from build123d import *

# Parameters (mm, degrees)
SKETCH2_R           = 45.212
SKETCH2_R_2         = 32.258
BOSS_EXTRUDE3_DEPTH = 40.64
SKETCH4_R           = 32.258
BOSS_EXTRUDE4_DEPTH = 7.62
BOSS_EXTRUDE4_TAPER = 25
CUT_EXTRUDE1_DEPTH  = 81.10791158
SKETCH7_R           = 2.286
CUT_EXTRUDE2_DEPTH  = 81.107911519
BOSS_EXTRUDE8_START = -7.62
BOSS_EXTRUDE8_DEPTH = 11.684
SKETCH18_R          = 8.567257543
CUT_EXTRUDE3_DEPTH  = 5.08
SKETCH19_R          = 2.286
CUT_EXTRUDE4_DEPTH  = 85.454467418
BOSS_EXTRUDE9_START = -15.24
BOSS_EXTRUDE9_DEPTH = 15.24
CUT_EXTRUDE5_START  = -28.956
SKETCH21_R          = 2.286
CUT_EXTRUDE5_DEPTH  = 28.956
CIRPATTERN1_COUNT   = 2


with BuildPart() as part:
    # Sketch2 → Boss-Extrude3 (new body)
    # profile 1 of 2: a face of its own
    with BuildSketch(Plane(origin=(0, 0, 0), x_dir=(1, 0, 0), z_dir=(0, 1, 0))):
        with Locations(Location((0, 0, 0), (0, 0, 270))):
            Circle(SKETCH2_R)
        Circle(SKETCH2_R_2, mode=Mode.SUBTRACT)
    # profile 2 of 2: a face of its own
    with BuildSketch(Plane(origin=(0, 0, 0), x_dir=(1, 0, 0), z_dir=(0, 1, 0))):
        Circle(SKETCH2_R_2)
        Polygon((0, 6.35), (-6.35, 3.483506942), (-6.35, -3.483506942), (0, -6.35), (6.35, -3.483506942), (6.35, 3.483506942), align=None, mode=Mode.SUBTRACT)
    extrude(amount=-BOSS_EXTRUDE3_DEPTH)

    # Sketch4 → Boss-Extrude4 (add)
    with BuildSketch(Plane(origin=(0, 0, 0), x_dir=(1, 0, 0), z_dir=(0, 1, 0))):
        Circle(SKETCH4_R)
    extrude(amount=BOSS_EXTRUDE4_DEPTH, taper=BOSS_EXTRUDE4_TAPER)

    # Sketch6 → Cut-Extrude1 (cut, through all)
    with BuildSketch(Plane(origin=(0, -40.64, 0), x_dir=(-1, 0, 0), z_dir=(0, -1, 0))):
        Polygon((6.35, -3.483506942), (0, -6.35), (-6.35, -3.483506942), (-6.35, 3.483506942), (0, 6.35), (6.35, 3.483506942), align=None)
    extrude(amount=-CUT_EXTRUDE1_DEPTH, mode=Mode.SUBTRACT)

    # Sketch7 → Cut-Extrude2 (cut, through all)
    with BuildSketch(Plane(origin=(0, 7.62, 0), x_dir=(1, 0, 0), z_dir=(0, 1, 0))):
        with Locations(Location((-16.495222192, 16.6624, 0), (0, 0, 270))):
            Circle(SKETCH7_R)
        with Locations(Location((16.6624, 16.6624, 0), (0, 0, 270))):
            Circle(SKETCH7_R)
        with Locations(Location((16.6624, -16.6624, 0), (0, 0, 270))):
            Circle(SKETCH7_R)
        with Locations(Location((-16.495222192, -16.6624, 0), (0, 0, 270))):
            Circle(SKETCH7_R)
    extrude(amount=-CUT_EXTRUDE2_DEPTH, mode=Mode.SUBTRACT)

    # Sketch12 → Boss-Extrude8 (add)
    with BuildSketch(Plane(origin=(0, 7.62, 0), x_dir=(1, 0, 0), z_dir=(0, 1, 0)).offset(BOSS_EXTRUDE8_START)):
        with BuildLine():
            ThreePointArc((-45.091998917, -3.291895759), (-45.888251869, -5.330050438), (-47.973633707, -5.992829324))
            ThreePointArc((-47.973633707, -5.992829324), (-61.102572974, -22.2395178), (-40.602051954, -26.246083736))
            ThreePointArc((-40.602051954, -26.246083736), (-38.578530729, -25.413344212), (-36.658465006, -26.462839746))
            ThreePointArc((-36.658465006, -26.462839746), (-42.485382771, -15.46341472), (-45.091998917, -3.291895759))
        make_face()
    extrude(amount=-BOSS_EXTRUDE8_DEPTH)

    # Sketch18 → Cut-Extrude3 (cut)
    with BuildSketch(Plane(origin=(0, 0, 0), x_dir=(1, 0, 0), z_dir=(0, 1, 0))):
        with Locations(Location((-49.645840541, -18.069608212, 0), (0, 0, 270))):
            Circle(SKETCH18_R)
    extrude(amount=-CUT_EXTRUDE3_DEPTH, mode=Mode.SUBTRACT)

    # Sketch19 → Cut-Extrude4 (cut, through all)
    with BuildSketch(Plane(origin=(0, -5.08, 0), x_dir=(1, 0, 0), z_dir=(0, 1, 0))):
        with Locations(Location((-49.645840541, -18.069608212, 0), (0, 0, 270))):
            Circle(SKETCH19_R)
    extrude(amount=-CUT_EXTRUDE4_DEPTH, mode=Mode.SUBTRACT)

    # Sketch20 → Boss-Extrude9 (add)
    with BuildSketch(Plane.XZ.offset(40.64).offset(BOSS_EXTRUDE9_START)):
        with BuildLine():
            ThreePointArc((42.485382852, -15.463414497), (44.831385262, -12.89196184), (48.307822394, -12.717373918))
            Line((48.307822394, -12.717373918), (61.237093085, -17.295868799))
            Line((61.237093085, -17.295868799), (62.000175566, -15.140990351))
            Line((62.000175566, -15.140990351), (60.601893265, -12.209430544))
            Line((60.601893265, -12.209430544), (44.72934622, -6.588666841))
            ThreePointArc((44.72934622, -6.588666841), (43.832551012, -11.082978649), (42.485382852, -15.463414497))
        make_face()
        with BuildLine():
            ThreePointArc((45.180509286, -21.309596065), (42.629626793, -18.941243028), (42.485382852, -15.463414497))
            ThreePointArc((42.485382852, -15.463414497), (40.701683588, -19.684966271), (38.499780526, -23.704257918))
            Line((38.499780526, -23.704257918), (54.271814253, -29.601179693))
            Line((54.271814253, -29.601179693), (57.22733096, -28.254273131))
            Line((57.22733096, -28.254273131), (58.027905034, -26.113040506))
            Line((58.027905034, -26.113040506), (45.180509286, -21.309596065))
        make_face()
    extrude(amount=BOSS_EXTRUDE9_DEPTH)

    # Sketch21 → Cut-Extrude5 (cut)
    # profile 1 of 2: a face of its own
    with BuildSketch(Plane.XZ.offset(40.64).offset(CUT_EXTRUDE5_START)):
        with BuildLine():
            Line((-20.08732464, 27.438707345), (-28.082012675, 35.43339538))
            ThreePointArc((-28.082012675, 35.43339538), (-31.885487137, 32.053715136), (-35.285134805, 28.268077504))
            Line((-35.285134805, 28.268077504), (-27.271504992, 20.254502449))
            Line((-27.271504992, 20.254502449), (-30.86360744, 16.662375455))
            Line((-30.86360744, 16.662375455), (-23.679427089, 9.478195103))
            ThreePointArc((-23.679427089, 9.478195103), (-9.311017295, 9.478195103), (-9.311017295, 23.846604897))
            Line((-9.311017295, 23.846604897), (-16.495222192, 31.030809794))
            Line((-16.495222192, 31.030809794), (-20.08732464, 27.438707345))
        make_face()
        with Locations(Location((-16.495222192, 16.6624, 0), (0, 0, 90))):
            Circle(SKETCH21_R, mode=Mode.SUBTRACT)
    # profile 2 of 2: a face of its own
    with BuildSketch(Plane.XZ.offset(40.64).offset(CUT_EXTRUDE5_START)):
        with BuildLine():
            ThreePointArc((16.6624, 26.8224), (6.5024, 16.6624), (16.6624, 6.5024))
            Line((16.6624, 6.5024), (26.8224, 6.5024))
            Line((26.8224, 6.5024), (26.8224, 11.844066963))
            Line((26.8224, 11.844066963), (43.63304965, 11.844066963))
            ThreePointArc((43.63304965, 11.844066963), (41.873887087, 17.050000709), (39.496151472, 22.004066963))
            Line((39.496151472, 22.004066963), (25.304864582, 22.004066963))
            Line((25.304864582, 22.004066963), (25.304864582, 26.8224))
            Line((25.304864582, 26.8224), (16.6624, 26.8224))
        make_face()
        with Locations(Location((16.6624, 16.6624, 0), (0, 0, 90))):
            Circle(SKETCH21_R, mode=Mode.SUBTRACT)
    cut_extrude5 = extrude(amount=CUT_EXTRUDE5_DEPTH, mode=Mode.SUBTRACT)

    # CirPattern1: Cut-Extrude5 ×2 about axis
    cirpattern1_axis = Axis((0, 0, 0), (0, 1, 0))
    for i in range(1, CIRPATTERN1_COUNT):
        add(cut_extrude5.rotate(cirpattern1_axis, i * 360 / CIRPATTERN1_COUNT), mode=Mode.SUBTRACT)


solid = part.part
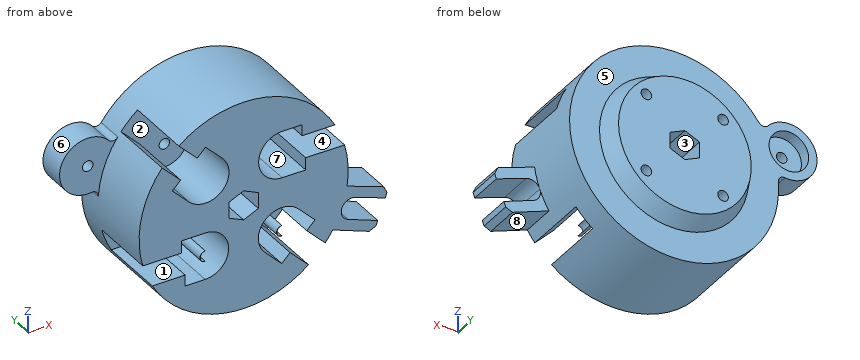
The listing builds one solid part. Answer for the finished solid, in the listing's coordinates (mm). Face numbers are marked on the shaded views. A direction names the side the tool comes from. Round coordinates to 2 decimals unless told otherwise and drop trailing zeros. Use a Markdown table: item, result. Add a question column.
1. For a pull along Z with two mould halves and no side action, classify the marked faces 5, 6, 7 and 8 as +Z half, -Z half, draft (parallel to the pull), parting line (faces both ways), or undercut.
2. A tool of negligible diameter and unlimited length cuts with its end or side. For the marked faces 1, 2, 3 and 4, from which of +Z, -Z, +X, -X, +Y, -Y can it reach the whole face along a straight path? Write none if from no direction.
3. Flat-ended cylindrical pins translate along their axes: P1, Ø4, axis at x = -32.5, y = -27, coming from the -Z side; P2, Ø5, axis at x = 48, y = -4, coming from the -Z side; P3, Ø15.5, axis at x = -49.65, z = 18.07, coming from the +Y side; P4, Ø2, axis at x = -3.5, y = -28, coming from the +Z side. Find the tip coordinate at first contact, or state that the pin passes through.
4. Consider line 1 (Z direction, x = 11, y = -20); line 2 (Z direction, x = -16.5, y = 4.5); line 3 (X direction, y = -4, z = -15). Determine where each line is inside the solid, lowest interval first.
5. The part is cut by section A-A (y = -38). Give the number of separate pieces and of enclosed holes in the cut face, and give its area (3 significant figures).
Reported:
| question | item | result |
|---|---|---|
| 1 | face 5 | draft |
| 1 | face 6 | parting line |
| 1 | face 7 | undercut |
| 1 | face 8 | -Z half |
| 2 | face 1 | -X, -Y |
| 2 | face 2 | -Y |
| 2 | face 3 | +Y, -Y |
| 2 | face 4 | +X, -Y |
| 3 | P1 | z = -33.37 |
| 3 | P2 | through |
| 3 | P3 | y = -5.08 |
| 3 | P4 | z = 45.14 |
| 4 | line 1 | -43.85 to -25.54, -8.12 to 8.23, 25.1 to 43.85 |
| 4 | line 2 | -25.25 to -18.95, -14.38 to 14.38, 18.95 to 25.25 |
| 4 | line 3 | -42.65 to -18.06, -14.93 to 15.09, 18.23 to 42.65 |
| 5 | separate pieces | 3 |
| 5 | enclosed holes | 1 |
| 5 | area | 4,480 mm^2 |
